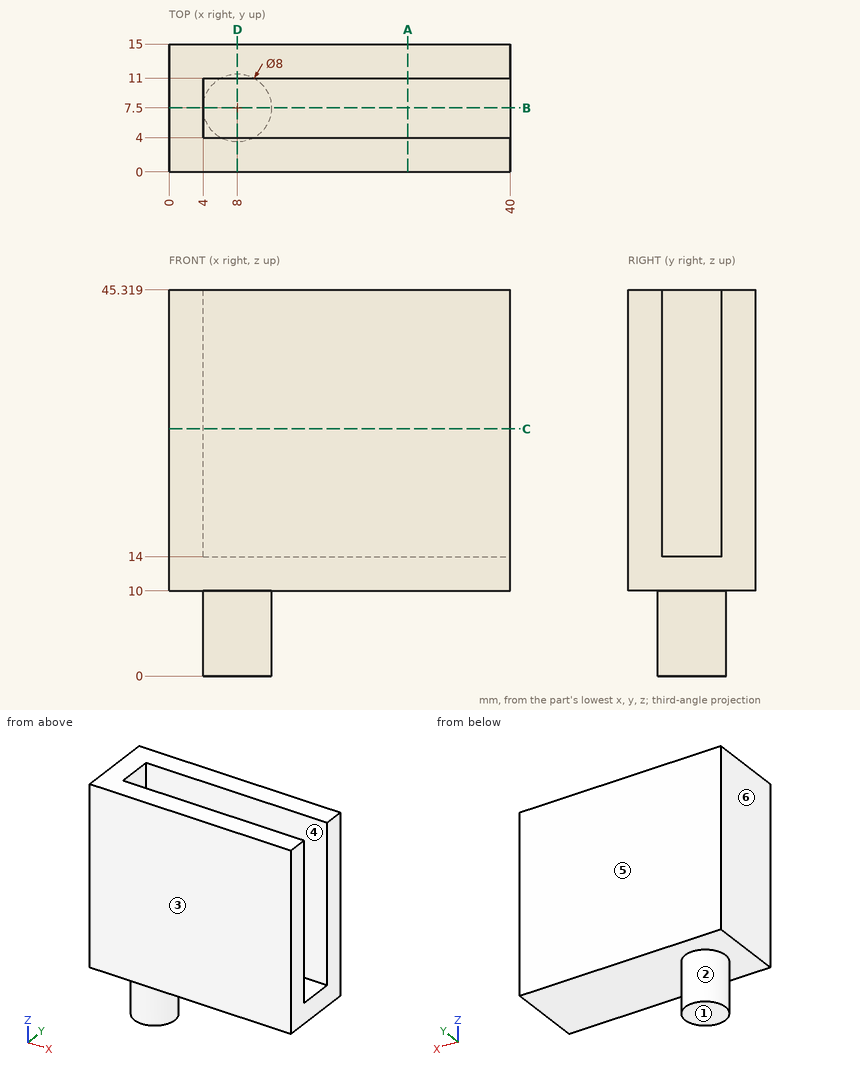
Check sheet for the drawn part. Datum: minimum x, y, z corner. Units: mm. A direction names the side the tool comes from. Coordinates: 2 decimals unless noted, no trailing zeros. Order: outer loops, then holes, each group sorted by start corner. A loop starts at its lowest first (then second) coordinate and runs counter-clockwise, first axis right, second up. Notation, with made-up numbers: M 43.25,35 L 82.25,35 A20 ccw 82.25,53 Z; hole C 65,51.25 d1. An arc over 180 degrees is marked long. One line per item, written item: value. Start each with the question number.
Item 1: Sectioned sample at D-D (x = 8). Enter the section's corners in (y, z).
Item 2: Mould release check, pull along Y, two halves, no side actions. Record for the marked faces 3, 4, 5 and 6: released by +Y, released by -Y, zero draft, split by the parting line, or undercut.
Item 3: Access from +Z, -Z, +X, -X, +Y, -Y to the whole of each face (thin tool, end or side, straight path). Record for the marked faces 1 and 2.
Item 4: Sectioned sample at B-B (y = 7.5). Enter the section's corners in (x, z), then the cut area to 3 significant figures.
Item 5: Sectioned sample at A-A (x = 28). Enter the section's corners in (y, z).
Item 6: Sectioned sample at C-C (z = 29). Enter the section's corners in (x, y).
Item 7: Gauge pin test, flat ends, axial feed: pin 1 (3.5 mm diameter, centred on x = 17, y = 6, fed in from +Z); pin 2 (5 mm diameter, centred on x = 19, y = 3, fed in from -Z); pin 3 (1.5 mm diameter, centred on y = 8, z = 34, fed in from +X). Record the tip position at first contact, or that the pin passes through.
Item 8: Scan lines: probe 1 along Y at (x, z) = (28.5, 38.5); probe 2 along Z at (x, y) = (6, 8.75); probe 3 along X at (y, z) = (6.5, 33). Record each from-to range of solid material in increasing order.
Conclusion:
1. outline: M 0,10 L 3.5,10 L 3.5,0 L 11.5,0 L 11.5,10 L 15,10 L 15,45.32 L 11,45.32 L 11,14 L 4,14 L 4,45.32 L 0,45.32 Z
2. face 3: released by -Y
2. face 4: undercut
2. face 5: released by +Y
2. face 6: zero draft
3. face 1: -Z, +X, -X, +Y, -Y
3. face 2: -Z
4. outline: M 0,10 L 4,10 L 4,0 L 12,0 L 12,10 L 40,10 L 40,14 L 4,14 L 4,45.32 L 0,45.32 Z
4. area: 365 mm^2
5. outline: M 0,10 L 15,10 L 15,45.32 L 11,45.32 L 11,14 L 4,14 L 4,45.32 L 0,45.32 Z
6. outline: M 0,0 L 40,0 L 40,4 L 4,4 L 4,11 L 40,11 L 40,15 L 0,15 Z
7. pin 1: stops at z = 14
7. pin 2: stops at z = 10
7. pin 3: stops at x = 4
8. probe 1: y = 0 to 4, 11 to 15
8. probe 2: z = 0 to 14
8. probe 3: x = 0 to 4
